Autodesk Inventor part; units mm, degrees
ref_plane "YZ Plane" through (0, 0, 0) normal (1, 0, 0) x (0, 1, 0)
ref_plane "XZ Plane" through (0, 0, 0) normal (0, 1, 0) x (-1, 0, 0)
ref_plane "XY Plane" through (0, 0, 0) normal (0, 0, 1) x (1, 0, 0)
sketch "Sketch1" plane through (0, 0, 0) normal (0, 1, 0) x (-1, 0, 0)
  arc A0 (-10.6066, -130.6066) -> (10.6066, -109.3934) centre (0, -120) ccw
  arc A1 (10.6066, -10.6066) -> (-10.6066, 10.6066) centre (0, 0) ccw
  arc A2 (-130.6066, -109.3934) -> (-109.3934, -130.6066) centre (-120, -120) ccw
  arc A3 (-109.3934, 10.6066) -> (-130.6066, -10.6066) centre (-120, 0) ccw
  arc A4 (10.6066, -10.6066) -> (10.6066, -109.3934) centre (120.3122, -60) ccw
  arc A5 (-10.6066, -130.6066) -> (-109.3934, -130.6066) centre (-60, -240.3122) ccw
  arc A6 (-109.3934, 10.6066) -> (-10.6066, 10.6066) centre (-60, 120.3122) ccw
  arc A7 (-130.6066, -109.3934) -> (-130.6066, -10.6066) centre (-244.217, -60) ccw
  circle A8 centre (7.1, 0) radius 1
  circle A9 centre (0, 7.1) radius 1
  circle A10 centre (-7.1, 0) radius 1
  circle A11 centre (0, -7.1) radius 1
  circle A12 centre (0, 0) radius 1.5
  circle A13 centre (-120, 0) radius 1.5
  circle A14 centre (-120, -120) radius 1.5
  circle A15 centre (0, -120) radius 1.5
  circle A16 centre (-120, 7.1) radius 1
  circle A17 centre (-127.1, 0) radius 1
  circle A18 centre (-120, -7.1) radius 1
  circle A19 centre (-112.9, 0) radius 1
  circle A20 centre (-127.1, -120) radius 1
  circle A21 centre (-120, -127.1) radius 1
  circle A22 centre (-112.9, -120) radius 1
  circle A23 centre (-120, -112.9) radius 1
  circle A24 centre (0, -127.1) radius 1
  circle A25 centre (7.1, -120) radius 1
  circle A26 centre (0, -112.9) radius 1
  circle A27 centre (-7.1, -120) radius 1
  line L0 (-21.7145, -8.1452) -> (-8.412, -21.4477)
  line L1 (-8.412, -21.4477) -> (-11.768, -24.8037)
  line L2 (-11.768, -24.8037) -> (-25.0705, -11.5012)
  line L3 (-25.0705, -11.5012) -> (-21.7145, -8.1452)
  line L4 (-95.1963, -11.768) -> (-108.4988, -25.0705)
  line L5 (-98.5523, -8.412) -> (-95.1963, -11.768)
  line L6 (-111.8548, -21.7145) -> (-98.5523, -8.412)
  line L7 (-108.4988, -25.0705) -> (-111.8548, -21.7145)
  line L8 (-108.232, -95.1963) -> (-94.9295, -108.4988)
  line L9 (-111.588, -98.5523) -> (-108.232, -95.1963)
  line L10 (-98.2855, -111.8548) -> (-111.588, -98.5523)
  line L11 (-94.9295, -108.4988) -> (-98.2855, -111.8548)
  line L12 (-24.8037, -108.232) -> (-11.5012, -94.9295)
  line L13 (-21.4477, -111.588) -> (-24.8037, -108.232)
  line L14 (-8.1452, -98.2855) -> (-21.4477, -111.588)
  line L15 (-11.5012, -94.9295) -> (-8.1452, -98.2855)
  circle A28 centre (-108.232, -60) radius 5
  line L16 (-9.5012, -49.1193) -> (-13.5012, -49.1193)
  line L17 (-13.5012, -49.1193) -> (-13.5012, -70.8807)
  line L18 (-13.5012, -70.8807) -> (-9.5012, -70.8807)
  line L19 (-9.5012, -70.8807) -> (-9.5012, -49.1193)
  line L20 (-9.5012, -49.1193) -> (-13.5012, -70.8807) construction
  line L21 (-13.5012, -49.1193) -> (-9.5012, -70.8807) construction
  circle A29 centre (-31.0935, -31.0935) radius 1.5
  circle A30 centre (-88.9065, -31.0935) radius 1.5
  circle A31 centre (-88.9065, -88.9065) radius 1.5
  circle A32 centre (-31.0935, -88.9065) radius 1.5
  point P0 (-60, -60)
  point P1 (-11.5012, -60)
  dimension "d13" = 360
  dimension "d19" = 360
  dimension "d23" = 360
  dimension "d29" = 360
  dimension "d31" = 10
  dimension "d32" = 4
  dimension "d33" = 3
  dimension "d36" = 360
  dimension "d48" = 57.813
extrude "Extrusion1" add sketch "Sketch1" along normal blind 3
sketch "Sketch2" plane through (0, 3, 0) normal (0, 1, 0) x (1, 0, 0)
  point P0 (0, 0)
sketch "Sketch3" plane through (0, 3, 0) normal (0, 1, 0) x (1, 0, 0)
  circle A0 centre (120, 120) radius 1.5
  arc A1 (-10.6066, 10.6066) -> (10.6066, -10.6066) centre (0, 0) ccw
  line L0 (-10.6066, -10.6066) -> (130.6066, 130.6066)
  arc A2 (130.6066, 109.3934) -> (109.3934, 130.6066) centre (120, 120) ccw
  arc A3 (109.3934, -10.6066) -> (130.6066, 10.6066) centre (120, 0) ccw
  line L1 (130.6066, -10.6066) -> (-10.6066, 130.6066)
  circle A4 centre (0, 0) radius 5
  line L2 (60, 60) -> (63.3779, 59.6927)
  circle A5 centre (120, 0) radius 5
  circle A6 centre (120, 120) radius 5
  circle A7 centre (0, 120) radius 5
  dimension "d41" = 10
  dimension "d44" = 360
sketch "Sketch4" plane through (0, 3, 0) normal (0, 1, 0) x (1, 0, 0)
  point P0 (0, 0)
extrude "Extrusion2" cut sketch "Sketch3" against normal blind 3 contours A0 L0 A6 | A0 L0 A6 | A5 L1 | L1 A5 | A4 L0 | L0 A4 | A7 L1 | L1 A7
properties part number "Base2"
The model under review builds one solid part; all positions refer to its coordinate system, in mm. Give positions to 0.01 mm unless a question says otherwise; leave off trailing zeros. Order: outer loops, then holes, each group sorted by start corner. A loop starts at its lowest first (then second) coordinate and runs counter-clockwise, first axis right, second up. Notation, with made-up numbers: M 7,-12 L 12,-12 A30 cw 12,22 Z; hole C 87,35 d9. An arc over 180 degrees is marked long. Answer in a Markdown table with one row per item. Add a question column.
1. Add section D-D on x = 83. State the section outline as (y, z) points.
2. Mouldability with a two-part tool opening along X and no side actions: class faces 1 (the cylindrical face through (120.336, 1.479, -59.289)), 2 (the flat face through (14.7, 1.48, -104.84)), 3 (the flat face through (61, 3, -59)) as released by +X, released by -X, zero draft, split by the parting line, or undercut.
3. Add section A-A on z = -60. State the section outline as (x, y) points.
4. For pin 1 Ø1.5 at (y, z) = (2, -64.5) entering from -X; pin 2 Ø5 at (x, z) = (31.09, -31.09) entering from +Y; pin 3 Ø1.2 at (x, z) = (0, 7.1) entering from +Y; pin 4 Ø0.9 at (y, z) = (1, -57) entering from +X, all flat-tipped, find the tip position at first contact; note any pin that passes through.
5. To check wall thickness, follow line 1 along Z through (x, y) = (32, 2.7); line 2 along X through (y, z) = (1.9, -11); line 3 along Z through (x, y) = (96, 2.95). State the ranges of each line that lie inside material, in increasing order.
6. Add section B-B on z = -105. State the section outline as (x, y) points, plus the area to 3 significant figures.
7. Add section C-C on y = 2.3. Count the separate pieces of the cut face and the enclosed holes in it, plus the area to 3 significant figures.
The answers:
| question | item | result |
|---|---|---|
| 1 | outline | M 0,-122.22 L 3,-122.22 L 3,2.22 L 0,2.22 Z |
| 2 | face 1 | released by +X |
| 2 | face 2 | undercut |
| 2 | face 3 | zero draft |
| 3 | outline | M 0,0 L 9.5,0 L 9.5,3 L 0,3 Z; M 13.5,0 L 103.23,0 L 103.23,3 L 13.5,3 Z; M 113.23,0 L 120.33,0 L 120.33,3 L 113.23,3 Z |
| 4 | pin 1 | x = -0.11 |
| 4 | pin 2 | y = 3 |
| 4 | pin 3 | through |
| 4 | pin 4 | x = 120.38 |
| 5 | line 1 | -123.3 to -90.1, -87.71 to -32.29, -29.9 to 3.3 |
| 5 | line 2 | -10.43 to 18.86, 24.57 to 95.96, 101.14 to 130.44 |
| 5 | line 3 | -125.51 to -109.57, -107.43 to -12.57, -10.96 to 5.51 |
| 6 | outline | M -8.73,0 L 14.86,0 L 14.86,3 L -8.73,3 Z; M 21.57,0 L 98.43,0 L 98.43,3 L 21.57,3 Z; M 105.14,0 L 128.8,0 L 128.8,3 L 105.14,3 Z |
| 6 | area | 372 mm2 |
| 7 | separate pieces | 1 |
| 7 | enclosed holes | 30 |
| 7 | area | 16,700 mm2 |
